from build123d import *

# Parameters (mm, degrees)
BOSS_EXTRUDE1_DEPTH      = 75
BOSS_EXTRUDE1_DEPTH_BACK = 75
SKETCH1_R                = 15.858479127
SKETCH1_R_2              = 14
SKETCH12_R               = 16
SKETCH12_R_2             = 14
BOSS_EXTRUDE2_DEPTH      = 80
SKETCH13_R               = 14
CUT_EXTRUDE1_DEPTH       = 81
CUT_EXTRUDE2_DEPTH       = 90
CUT_EXTRUDE2_DEPTH_BACK  = 95
SKETCH15_R               = 14


with BuildPart() as part:
    # Sketch1 → Boss-Extrude1 (new, two sides: drawn at the far end of the back side and taken through both)
    with BuildSketch(Plane.XY.offset(-BOSS_EXTRUDE1_DEPTH_BACK)):
        Circle(SKETCH1_R)
        Circle(SKETCH1_R_2, mode=Mode.SUBTRACT)
    extrude(amount=BOSS_EXTRUDE1_DEPTH + BOSS_EXTRUDE1_DEPTH_BACK)

    # Sketch2 → Revolve1 (revolve)
    with BuildSketch(Plane(origin=(0, 0, 0), x_dir=(0, 0, -1), z_dir=(1, 0, 0)), mode=Mode.PRIVATE) as revolve1_sk:
        Polygon((75, 15.858479127), (72, 15.858479127), (72, 17.358479127), align=None)
    revolve(revolve1_sk.sketch.rotate(Axis((0, 0, 0), (0, 0, -1)), 90), axis=Axis((0, 0, 0), (0, 0, -1)))

    # Sketch3 → Revolve2 (revolve)
    with BuildSketch(Plane(origin=(0, 0, 0), x_dir=(0, 0, -1), z_dir=(1, 0, 0)), mode=Mode.PRIVATE) as revolve2_sk:
        Polygon((72, 15.858479127), (69.040504624, 15.858479127), (69.040504624, 17.393237669), align=None)
    revolve(revolve2_sk.sketch.rotate(Axis((0, 0, 0), (0, 0, -1)), 90), axis=Axis((0, 0, 0), (0, 0, -1)))

    # Sketch4 → Revolve3 (revolve)
    with BuildSketch(Plane(origin=(0, 0, 0), x_dir=(0, 0, -1), z_dir=(1, 0, 0)), mode=Mode.PRIVATE) as revolve3_sk:
        Polygon((69.040504624, 15.858479127), (66.023310335, 15.858479127), (66.023310335, 17.393237669), align=None)
    revolve(revolve3_sk.sketch.rotate(Axis((0, 0, 0), (0, 0, -1)), 90), axis=Axis((0, 0, 0), (0, 0, -1)))

    # Sketch5 → Revolve4 (revolve)
    with BuildSketch(Plane(origin=(0, 0, 0), x_dir=(0, 0, -1), z_dir=(1, 0, 0)), mode=Mode.PRIVATE) as revolve4_sk:
        Polygon((66.023310335, 15.858479127), (63.006116045, 15.858479127), (63.006116045, 17.393237669), align=None)
    revolve(revolve4_sk.sketch.rotate(Axis((0, 0, 0), (0, 0, -1)), 90), axis=Axis((0, 0, 0), (0, 0, -1)))

    # Sketch6 → Revolve5 (revolve)
    with BuildSketch(Plane(origin=(0, 0, 0), x_dir=(0, 0, -1), z_dir=(1, 0, 0)), mode=Mode.PRIVATE) as revolve5_sk:
        Polygon((63.006116045, 15.858479127), (59.988921756, 15.858479127), (59.988921756, 17.393237669), align=None)
    revolve(revolve5_sk.sketch.rotate(Axis((0, 0, 0), (0, 0, -1)), 90), axis=Axis((0, 0, 0), (0, 0, -1)))

    # Sketch7 → Revolve6 (revolve)
    with BuildSketch(Plane(origin=(0, 0, 0), x_dir=(0, 0, -1), z_dir=(1, 0, 0)), mode=Mode.PRIVATE) as revolve6_sk:
        Polygon((-75, 15.858479127), (-72, 15.858479127), (-72, 17.393237669), align=None)
    revolve(revolve6_sk.sketch.rotate(Axis((0, 0, 0), (0, 0, -1)), 90), axis=Axis((0, 0, 0), (0, 0, -1)))

    # Sketch8 → Revolve7 (revolve)
    with BuildSketch(Plane(origin=(0, 0, 0), x_dir=(0, 0, -1), z_dir=(1, 0, 0)), mode=Mode.PRIVATE) as revolve7_sk:
        Polygon((-72, 15.858479127), (-69.040504624, 15.858479127), (-69.040504624, 17.393237669), align=None)
    revolve(revolve7_sk.sketch.rotate(Axis((0, 0, 0), (0, 0, -1)), 90), axis=Axis((0, 0, 0), (0, 0, -1)))

    # Sketch9 → Revolve8 (revolve)
    with BuildSketch(Plane(origin=(0, 0, 0), x_dir=(0, 0, -1), z_dir=(1, 0, 0)), mode=Mode.PRIVATE) as revolve8_sk:
        Polygon((-69.040504624, 15.858479127), (-66.023310335, 15.858479127), (-66.023310335, 17.393237669), align=None)
    revolve(revolve8_sk.sketch.rotate(Axis((0, 0, 0), (0, 0, -1)), 90), axis=Axis((0, 0, 0), (0, 0, -1)))

    # Sketch10 → Revolve9 (revolve)
    with BuildSketch(Plane(origin=(0, 0, 0), x_dir=(0, 0, -1), z_dir=(1, 0, 0)), mode=Mode.PRIVATE) as revolve9_sk:
        Polygon((-66.023310335, 15.858479127), (-63.006116045, 15.858479127), (-63.006116045, 17.393237669), align=None)
    revolve(revolve9_sk.sketch.rotate(Axis((0, 0, 0), (0, 0, -1)), 90), axis=Axis((0, 0, 0), (0, 0, -1)))

    # Sketch11 → Revolve10 (revolve)
    with BuildSketch(Plane(origin=(0, 0, 0), x_dir=(0, 0, -1), z_dir=(1, 0, 0)), mode=Mode.PRIVATE) as revolve10_sk:
        Polygon((-63.006116045, 15.858479127), (-59.988921756, 15.858479127), (-59.988921756, 17.393237669), align=None)
    revolve(revolve10_sk.sketch.rotate(Axis((0, 0, 0), (0, 0, 1)), 270), axis=Axis((0, 0, 0), (0, 0, 1)))

    # Sketch12 → Boss-Extrude2 (add)
    with BuildSketch(Plane(origin=(0, 0, 0), x_dir=(0, 0, -1), z_dir=(1, 0, 0))):
        Circle(SKETCH12_R)
        Circle(SKETCH12_R_2, mode=Mode.SUBTRACT)
    extrude(amount=BOSS_EXTRUDE2_DEPTH)

    # Sketch13 → Cut-Extrude1 (cut)
    with BuildSketch(Plane(origin=(0, 0, 0), x_dir=(0, 0, -1), z_dir=(1, 0, 0))):
        with Locations(Location((0, 0, 0), (0, 0, 90))):
            Circle(SKETCH13_R)
    extrude(amount=CUT_EXTRUDE1_DEPTH, mode=Mode.SUBTRACT)

    # Sketch15 → Cut-Extrude2 (cut, two sides: drawn at the far end of the back side and taken through both)
    with BuildSketch(Plane.XY.offset(-CUT_EXTRUDE2_DEPTH_BACK)):
        Circle(SKETCH15_R)
    extrude(amount=CUT_EXTRUDE2_DEPTH + CUT_EXTRUDE2_DEPTH_BACK, mode=Mode.SUBTRACT)

    # Sketch16 → Revolve11 (revolve)
    with BuildSketch(Plane.XY, mode=Mode.PRIVATE) as revolve11_sk:
        Polygon((80, 16), (77.013377654, 16), (77.013377654, 17.472012137), align=None)
    revolve(revolve11_sk.sketch.rotate(Axis((0, 0, 0), (-1, 0, 0)), 90), axis=Axis((0, 0, 0), (-1, 0, 0)))

    # Sketch17 → Revolve12 (revolve)
    with BuildSketch(Plane.XY, mode=Mode.PRIVATE) as revolve12_sk:
        Polygon((77.013377654, 16), (74.024743999, 16), (74.024743999, 17.472012137), align=None)
    revolve(revolve12_sk.sketch.rotate(Axis((0, 0, 0), (-1, 0, 0)), 90), axis=Axis((0, 0, 0), (-1, 0, 0)))

    # Sketch18 → Revolve13 (revolve)
    with BuildSketch(Plane.XY, mode=Mode.PRIVATE) as revolve13_sk:
        Polygon((74.024743999, 16), (71.036110344, 16), (71.036110344, 17.472012137), align=None)
    revolve(revolve13_sk.sketch.rotate(Axis((0, 0, 0), (-1, 0, 0)), 90), axis=Axis((0, 0, 0), (-1, 0, 0)))

    # Sketch19 → Revolve14 (revolve)
    with BuildSketch(Plane.XY, mode=Mode.PRIVATE) as revolve14_sk:
        Polygon((71.036110344, 16), (68.047476689, 16), (68.047476689, 17.472012137), align=None)
    revolve(revolve14_sk.sketch.rotate(Axis((0, 0, 0), (-1, 0, 0)), 90), axis=Axis((0, 0, 0), (-1, 0, 0)))

    # Sketch20 → Revolve15 (revolve)
    with BuildSketch(Plane.XY, mode=Mode.PRIVATE) as revolve15_sk:
        Polygon((68.047476689, 16), (65.058843034, 16), (65.058843034, 17.472012137), align=None)
    revolve(revolve15_sk.sketch.rotate(Axis((0, 0, 0), (-1, 0, 0)), 90), axis=Axis((0, 0, 0), (-1, 0, 0)))


solid = part.part
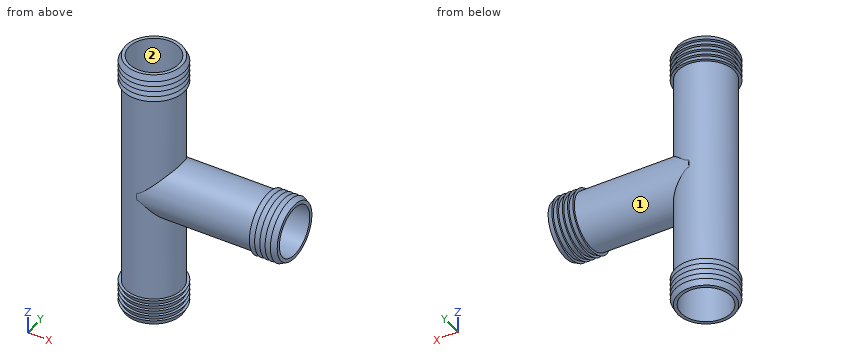
Input: part model. Units: mm. Frame: model coordinates. Face numbers are marked on the shaded views. A direction names the side the tool comes from. Coordinates: 2 decimals unless noted, no trailing zeros. Order: outer loops, then holes, each group sorted by start corner. A loop starts at its lowest first (then second) coordinate and runs counter-clockwise, first axis right, second up. Notation, with made-up numbers: M 29.5,10.25 L 44.5,10.25 A23 cw 44.5,40.25 Z; hole C 76.5,87 d10. An arc over 180 degrees is marked long. Write item = value, one per line. Start each with the question number.
(1) Section C-C on x = 38. Output: boundary loops of the cut face in (y, z).
(2) Reachability of the marked faces 1 and 2 from +Z, -Z, +X, -X, +Y, -Y: full face, straight path, thin tool, end or side. Return the list, or none.
(3) Section B-B on y = 0. Give the number of separate pieces and of enclosed holes in the cut face, and give its area (3 significant figures).
(4) Section D-D on z = 19.5. Output: boundary loops of the cut face in (x, y).
(5) Line query: line 1 along Y through (x, z) = (7, 0); line 2 along X through (y, z) = (-1, -32.5). Output: solid intervals per line, ascending. Write a range as [from, to].
(6) First-contact query: P1, Ø10.5, axis at y = -0.5, z = -3, coming from the -X side; P2, Ø12, axis at x = 48.5, y = 8, coming from the +Z side; P3, Ø17, axis at x = 0, y = 0, coming from the -Z side; P4, Ø3, axis at y = -7.5, z = 13.5, coming from the -X side. Flat tips, straight axial feed; report the tip coordinate or a pass-through.
Result set:
q1.outline = C 0,0 d32; hole C 0,0 d28
q2.face_1 = none
q2.face_2 = +Z, -Z
q3.separate_pieces = 3
q3.enclosed_holes = 0
q3.area = 830 mm²
q4.outline = C 0,0 d31.72; hole C 0,0 d28
q5.line_1 = [-16, -14], [14, 16]
q5.line_2 = [-15.83, -13.96], [13.96, 15.83]
q6.P1 = -15.86
q6.P2 = 15.87
q6.P3 = through
q6.P4 = -14.68
